Here's how the part is built. I have some questions about the finished solid (model axes, mm). A direction names the side the tool comes from. Coordinates: 2 decimals unless noted, no trailing zeros. Write each loop counter-clockwise with the first axis right and the second up, starting at its lowest first coordinate (ties: lowest second). Pieces come first, ordered by that corner, then holes. Notation, with made-up numbers: (86.25, 24) -> (110.25, 24) arc R29 cw to (110.25, 45) -> close; hole circle Ø3 at (67.5, 88). An arc over 180 degrees is marked (long way). Use a Markdown table: item, result. Add a question column.
Item 1: If I drill on line 1 along Z through (x, y) = (-113.35, 234.5); line 2 along Y through (x, z) = (-111.5, 117); line 3 along Z through (x, y) = (-112.8, 215.5), over which ranges is the centre line in solid material (lowest first)? Write a range as from..to.
Item 2: Imagine slicing it at B-B, the plane y = 218. Write out the boundary of the cut face in (x, z).
Item 3: On a 3-axis mill with a long thin cutter (end or side, diameter ignored), from which of +Z, -Z, +X, -X, +Y, -Y can I reach the whole of each face in a straight line? I mean faces 5 (the flat face through (-113, 235, 80.566)), 6 (the flat face through (-113, 228, 110.066)), 7 (the flat face through (-113, 227, 75.066)). Say none if no direction works.
Item 4: Imagine slicing it at C-C, the plane z = 112. Write out the boundary of the cut face in (x, y), and give its area (3 significant figures).
Item 5: Will these pins go through, and if not, where does the flat tip stop? pin 1 Ø2 at (y, z) = (205, 60) entering from -X; pin 2 Ø2.5 at (x, y) = (-113, 236) entering from +Z; pin 3 Ø2.5 at (x, y) = (-112.5, 226) entering from -Z; pin 4 Ø1.1 at (y, z) = (193.08, 65.57) entering from +X.
Item 6: Imagine slicing it at A-A, the plane x = -111.35. Count the separate pieces of the cut face and the enclosed holes in it, and give its area (3 significant figures).
Item 7: If we mould it in two halves opening along Y, with no side actions, what happens to faces 1 (the flat face through (-113, 240.331, 106)), 2 (the flat face through (-113, 142.581, 92)), 3 (the flat face through (-113, 212.581, 118)), 4 (the flat face through (-115.112, 178, 93))? For each: pulls with the +Y half, pulls with the -Y half, needs draft (parallel to the pull), parting line crosses it, or undercut.
```python
from build123d import *

# Parameters (mm, degrees)
BOSS_EXTRUDE1_DEPTH = 5.000002682
SKETCH2_R           = 2.000000134
CUT_EXTRUDE1_DEPTH  = 251.578832691
SKETCH3_R           = 2.000006516
CUT_EXTRUDE2_DEPTH  = 251.578832691
SKETCH4_R           = 0.899997723
CUT_EXTRUDE3_DEPTH  = 2.999998629
SKETCH5_R           = 0.899983627
CUT_EXTRUDE4_DEPTH  = 3.00000608
SKETCH6_R           = 0.900000334
CUT_EXTRUDE5_DEPTH  = 3.00000608
SKETCH7_R           = 0.899990272
CUT_EXTRUDE6_DEPTH  = 2.999998629
SKETCH8_R           = 0.899993205
CUT_EXTRUDE7_DEPTH  = 3.00000608
SKETCH9_R           = 0.899993205
CUT_EXTRUDE8_DEPTH  = 3.00000608
SKETCH10_R          = 0.899997723
CUT_EXTRUDE9_DEPTH  = 2.999998629
SKETCH11_R          = 0.899993205
CUT_EXTRUDE10_DEPTH = 2.999998629
SKETCH12_W          = 2.2
SKETCH12_H          = 11.5
BOSS_EXTRUDE2_DEPTH = 5


with BuildPart() as part:
    # Sketch1 → Boss-Extrude1 (new body)
    with BuildSketch(Plane(origin=(-115.112178028, 0, 0), x_dir=(0, -1, 0), z_dir=(-1, 0, 0))):
        Polygon((-142.581447959, 52.566498518), (-142.581447959, 132.56649673), (-210.581451654, 132.56649673), (-210.866093636, 132.546141744), (-211.144909263, 132.485494018), (-211.412280798, 132.385760546), (-211.662739515, 132.249012589), (-211.891174316, 132.078006864), (-212.09295094, 131.876215339), (-212.263956666, 131.647780538), (-212.400704622, 131.39732182), (-212.500438094, 131.129965186), (-212.561100721, 130.851134658), (-212.581455708, 130.566492677), (-212.581455708, 54.566498846), (-212.561100721, 54.281868041), (-212.500438094, 54.003033787), (-212.400704622, 53.735669702), (-212.263956666, 53.485218436), (-212.09295094, 53.256779909), (-211.891174316, 53.05499956), (-211.662739515, 52.883990109), (-211.412280798, 52.747234702), (-211.144909263, 52.647516131), (-210.866093636, 52.586857229), (-210.581451654, 52.566498518), align=None)
    extrude(amount=-BOSS_EXTRUDE1_DEPTH)

    # Sketch2 → Cut-Extrude1 (cut, through all)
    with BuildSketch(Plane.ZY.offset(115.112178028)):
        with Locations((97.566500306, 147.581450641)):
            Circle(SKETCH2_R)
    extrude(amount=-CUT_EXTRUDE1_DEPTH, mode=Mode.SUBTRACT)

    # Sketch3 → Cut-Extrude2 (cut, through all)
    with BuildSketch(Plane(origin=(-110.112175345, 0, 0), x_dir=(0, 0, -1), z_dir=(1, 0, 0))):
        with Locations((-87.566494942, 147.581450641)):
            Circle(SKETCH3_R)
    extrude(amount=-CUT_EXTRUDE2_DEPTH, mode=Mode.SUBTRACT)

    # Sketch4 → Cut-Extrude3 (cut)
    with BuildSketch(Plane(origin=(-110.112175345, 0, 0), x_dir=(0, 0, -1), z_dir=(1, 0, 0))):
        with Locations((-119.566500187, 165.081456304)):
            Circle(SKETCH4_R)
    cut_extrude3 = extrude(amount=-CUT_EXTRUDE3_DEPTH, mode=Mode.SUBTRACT)

    # Sketch5 → Cut-Extrude4 (cut)
    with BuildSketch(Plane.ZY.offset(115.112178028)):
        with Locations((125.066503882, 160.081461072)):
            Circle(SKETCH5_R)
    extrude(amount=-CUT_EXTRUDE4_DEPTH, mode=Mode.SUBTRACT)

    # Sketch6 → Cut-Extrude5 (cut)
    with BuildSketch(Plane.ZY.offset(115.112178028)):
        with Locations((60.066498816, 160.081461072)):
            Circle(SKETCH6_R)
    extrude(amount=-CUT_EXTRUDE5_DEPTH, mode=Mode.SUBTRACT)

    # Sketch7 → Cut-Extrude6 (cut)
    with BuildSketch(Plane(origin=(-110.112175345, 0, 0), x_dir=(0, 0, -1), z_dir=(1, 0, 0))):
        with Locations((-67.566499114, 160.081461072)):
            Circle(SKETCH7_R)
    cut_extrude6 = extrude(amount=-CUT_EXTRUDE6_DEPTH, mode=Mode.SUBTRACT)

    # Sketch8 → Cut-Extrude7 (cut)
    with BuildSketch(Plane.ZY.offset(115.112178028)):
        with Locations((125.066503882, 205.08146286)):
            Circle(SKETCH8_R)
    extrude(amount=-CUT_EXTRUDE7_DEPTH, mode=Mode.SUBTRACT)

    # Sketch9 → Cut-Extrude8 (cut)
    with BuildSketch(Plane.ZY.offset(115.112178028)):
        with Locations((60.066498816, 205.08146286)):
            Circle(SKETCH9_R)
    extrude(amount=-CUT_EXTRUDE8_DEPTH, mode=Mode.SUBTRACT)

    # Sketch10 → Cut-Extrude9 (cut)
    with BuildSketch(Plane(origin=(-110.112175345, 0, 0), x_dir=(0, 0, -1), z_dir=(1, 0, 0))):
        with Locations((-119.566500187, 193.081453443)):
            Circle(SKETCH10_R)
    cut_extrude9 = extrude(amount=-CUT_EXTRUDE9_DEPTH, mode=Mode.SUBTRACT)

    # Sketch11 → Cut-Extrude10 (cut)
    with BuildSketch(Plane(origin=(-110.112175345, 0, 0), x_dir=(0, 0, -1), z_dir=(1, 0, 0))):
        with Locations((-67.566499114, 208.081454039)):
            Circle(SKETCH11_R)
    cut_extrude10 = extrude(amount=-CUT_EXTRUDE10_DEPTH, mode=Mode.SUBTRACT)

    # Sketch12 → Boss-Extrude2 (add)
    with BuildSketch(Plane(origin=(-110.112175345, 0, 0), x_dir=(0, 0, -1), z_dir=(1, 0, 0))):
        Polygon((-110.066497624, 226.581455708), (-110.066497624, 212.581455708), (-75.066497624, 212.581455708), (-75.066497624, 226.581455708), (-75.066497624, 242.581455708), (-110.066497624, 242.581455708), align=None)
        with Locations((-105.666497624, 234.581455708)):
            Rectangle(SKETCH12_W, SKETCH12_H, mode=Mode.SUBTRACT)
        with Locations((-79.466497624, 234.581455708)):
            Rectangle(SKETCH12_W, SKETCH12_H, mode=Mode.SUBTRACT)
    extrude(amount=-BOSS_EXTRUDE2_DEPTH)

    # Mirror1: Cut-Extrude3, Cut-Extrude6, Cut-Extrude9, Cut-Extrude10 across plane
    add(cut_extrude3.mirror(Plane.XY.offset(92.566497624)), mode=Mode.SUBTRACT)
    add(cut_extrude6.mirror(Plane.XY.offset(92.566497624)), mode=Mode.SUBTRACT)
    add(cut_extrude9.mirror(Plane.XY.offset(92.566497624)), mode=Mode.SUBTRACT)
    add(cut_extrude10.mirror(Plane.XY.offset(92.566497624)), mode=Mode.SUBTRACT)


solid = part.part
```
Ans:
| question | item | result |
|---|---|---|
| 1 | line 1 | z = 75.07..78.37, 80.57..104.57, 106.77..110.07 |
| 1 | line 2 | y = 142.58..159.38, 160.78..207.38, 208.78..212.58 |
| 1 | line 3 | z = 75.07..110.07 |
| 2 | outline | (-115.11, 75.07) -> (-110.11, 75.07) -> (-110.11, 110.07) -> (-115.11, 110.07) -> close |
| 3 | face 5 | +X, -X |
| 3 | face 6 | +Z, +X, -X, +Y |
| 3 | face 7 | -Z, +X, -X, +Y |
| 4 | outline | (-115.11, 142.58) -> (-110.11, 142.58) -> (-110.11, 212.58) -> (-115.11, 212.58) -> close |
| 4 | area | 350 mm^2 |
| 5 | pin 1 | stops at x = -115.11 |
| 5 | pin 2 | stops at z = 110.07 |
| 5 | pin 3 | stops at z = 75.07 |
| 5 | pin 4 | stops at x = -113.11 |
| 6 | separate pieces | 1 |
| 6 | enclosed holes | 12 |
| 6 | area | 6,550 mm^2 |
| 7 | face 1 | undercut |
| 7 | face 2 | pulls with the -Y half |
| 7 | face 3 | pulls with the +Y half |
| 7 | face 4 | needs draft |
